```python
from build123d import *

# Parameters (mm, degrees)
F0_W     = 254
F0_H     = 127
F1_DEPTH = 76.2
F1_TAPER = 30
F2_R     = 12.7
F4_DEPTH = 25.4


with BuildPart() as f1:
    # F0 (on Top) → F1 (new body)
    with BuildSketch(Plane.XY):
        Rectangle(F0_W, F0_H)
    extrude(amount=F1_DEPTH, taper=F1_TAPER)

    # F2
    f2_edges = [f1.edges().sort_by_distance(p)[0] for p in [
        (83.005909, 0, 76.2),
        (0, 19.505909, 76.2),
        (-83.005909, 0, 76.2),
        (0, -19.505909, 76.2),
        (105.002955, 41.502955, 38.1),
        (105.002955, -41.502955, 38.1),
        (-105.002955, -41.502955, 38.1),
        (-105.002955, 41.502955, 38.1),
    ]]
    fillet(f2_edges, radius=F2_R)

    # F3 (on face) → F4 (join)
    with BuildSketch(Plane.XY.offset(76.2)):
        with BuildLine():
            ThreePointArc((29.3234873591, -12.173561069), (31.1374631565, -6.2065198118), (31.75, 0))
            ThreePointArc((31.75, 0), (31.1374631565, 6.2065198118), (29.3234873591, 12.173561069))
            Line((29.3234873591, 12.173561069), (-29.3234873591, 12.173561069))
            ThreePointArc((-29.3234873591, 12.173561069), (-31.75, 0), (-29.3234873591, -12.173561069))
            Line((-29.3234873591, -12.173561069), (29.3234873591, -12.173561069))
        make_face()
    extrude(amount=F4_DEPTH)


solid = f1.part
```
Here's how the part is built. I have some questions about the finished solid (model axes, mm). A direction names the side the tool comes from. Give positions to 0.01 mm unless a question says otherwise; leave off trailing zeros. Loops run counter-clockwise (first coordinate to the right, second up) from the corner with the lowest first, then second, coordinate; pieces in that order, holes last. Notation, with made-up numbers: M 85,48.25 L 127,48.25 A25 ccw 127,74.25 Z; hole C 0.5,45.25 d6. An arc over 180 degrees is marked long. Use one line per item in the form item = value. Start each with the question number.
Q1. If we section it at A-A (x = -20): Write out the boundary of the cut face in (y, z).
Q2. If we section it at C-C (x = 56.5): Write out the boundary of the cut face in (y, z), then the cut area to 3 significant figures.
Q3. Which directions (+Z, -Z, +X, -X, +Y, -Y) give clear straight access to the entire face, cutting with the end or side of a thin tool? Please do faces 1 (the cylindrical face through (-31.75, 0.17, 88.72)), 2 (the flat face through (0, 12.174, 89)), 3 (the flat face through (0, -12.174, 89)).
Q4. I need wall thicknesses on line 1 along Y through (x, z) = (-42.5, 60); line 2 along Y through (x, z) = (56.5, 69); line 3 along X through (y, z) = (11, 23). Which ranges of each line are inside material? Lowest first, please.
Q5. Will these pins go through, and if not, where does the flat tip stop? pin 1 Ø12.5 at (x, z) = (-9.5, 82.5) entering from +Y; pin 2 Ø1.5 at (x, z) = (-29.5, 20.5) entering from +Y; pin 3 Ø10 at (y, z) = (-7.5, 81.5) entering from +X.
Q6. If we section it at B-B (z = 91): Write out the boundary of the cut face in (x, y), then the cut area to 3 significant figures.
Taken from the geometry:
q1.outline = M -63.5,0 L 63.5,0 L 23.17,69.85 A12.7 ccw 12.17,76.2 L 12.17,101.6 L -12.17,101.6 L -12.17,76.2 A12.7 ccw -23.17,69.85 Z
q2.outline = M -63.5,0 L 63.5,0 L 23.17,69.85 A12.7 ccw 12.17,76.2 L -12.17,76.2 A12.7 ccw -23.17,69.85 Z
q2.area = 6,310 mm^2
q3.face_1 = +Z, -X
q3.face_2 = +Z, +X, -X, +Y
q3.face_3 = +Z, +X, -X, -Y
q4.line_1 = -28.86 to 28.86
q4.line_2 = -23.66 to 23.66
q4.line_3 = -113.72 to 113.72
q5.pin_1 = 12.17
q5.pin_2 = 52.1
q5.pin_3 = 31.65
q6.outline = M -29.32,-12.17 L 29.32,-12.17 A31.75 ccw 29.32,12.17 L -29.32,12.17 A31.75 ccw Z
q6.area = 1,510 mm^2
